Design review of the part built by this model. Coordinates are the model's own, in mm. Face numbers are marked on the shaded views. A direction names the side the tool comes from. Coordinates: 2 decimals unless noted, no trailing zeros. Write each loop counter-clockwise with the first axis right and the second up, starting at its lowest first coordinate (ties: lowest second). Pieces come first, ordered by that corner, then holes. Notation, with made-up numbers: M 16,18.25 L 32,18.25 A28 cw 32,40.25 Z; hole C 46,21.25 d8. An arc over 180 degrees is marked long. Return JSON: item names as keys, results as strings. Group by question number.
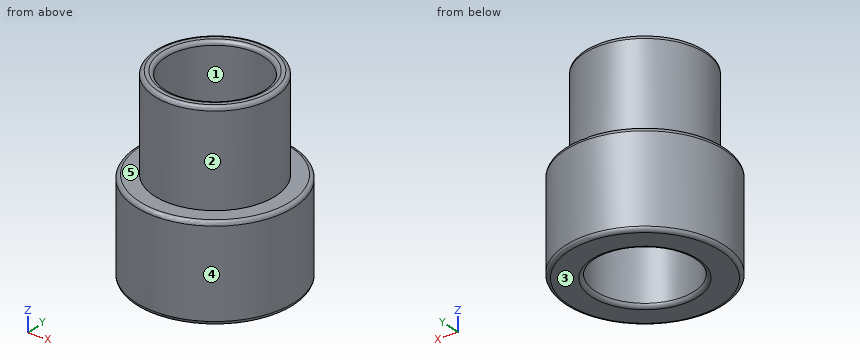
```python
from build123d import *

# Parameters (mm, degrees)
CYLINDER002_R     = 13
CYLINDER002_DEPTH = 120
CYLINDER001_R     = 16
CYLINDER001_DEPTH = 50
FILLET001_R       = 1
CYLINDER003_R     = 16
CYLINDER003_DEPTH = 120
CYLINDER_R        = 21
CYLINDER_DEPTH    = 25
FILLET_R          = 1


with BuildPart() as obj1:
    # Cylinder002 → Cylinder002 (new body)
    with BuildSketch(Plane.XY.offset(-60)):
        Circle(CYLINDER002_R)
    extrude(amount=CYLINDER002_DEPTH)


with BuildPart() as fillet001:
    # Cylinder001 → Cylinder001 (new body)
    with BuildSketch(Plane.XY):
        Circle(CYLINDER001_R)
    extrude(amount=CYLINDER001_DEPTH)

    # Cut: cut obj1
    add(obj1.part, mode=Mode.SUBTRACT)

    # Fillet001
    fillet001_edges = [fillet001.edges().sort_by_distance(p)[0] for p in [
        (-16, 0, 50),
        (-13, 0, 50),
        (-13, 0, 0),
    ]]
    fillet(fillet001_edges, radius=FILLET001_R)


with BuildPart() as obj2:
    # Cylinder003 → Cylinder003 (new body)
    with BuildSketch(Plane.XY.offset(-60)):
        Circle(CYLINDER003_R)
    extrude(amount=CYLINDER003_DEPTH)


with BuildPart() as fusion:
    # Cylinder → Cylinder (new body)
    with BuildSketch(Plane.XY):
        Circle(CYLINDER_R)
    extrude(amount=CYLINDER_DEPTH)

    # Cut001: cut obj2
    add(obj2.part, mode=Mode.SUBTRACT)

    # Fillet
    fillet_edges = [fusion.edges().sort_by_distance(p)[0] for p in [
        (-21, 0, 25),
        (-21, 0, 0),
    ]]
    fillet(fillet_edges, radius=FILLET_R)

    # Fusion: union Fillet001
    add(fillet001.part)


solid = fusion.part
```
Item 1: For pin 1 (4 mm diameter, centred on y = -11.5, z = 30.5, fed in from +X); pin 2 (12 mm diameter, centred on x = 2, y = 4, fed in from +Z); pin 3 (5 mm diameter, centred on x = -16.5, y = -15, fed in from +Z); pin 4 (1.5 mm diameter, centred on y = -1.5, z = 41, fed in from +X), all flat-tipped, find the tip position at first contact; note any pin that passes through.
Item 2: Add section A-A (x = 0). Write out the cut boundary in (y, z).
Item 3: Machinability: for the marked faces 4 and 5, which of the approach directions +Z, -Z, +X, -X, +Y, -Y give a long, thin tool a straight path to every point of the face, cutting with its end or side? Answer none if there is none.
Item 4: The part is to be moulded in two halves that separate along Y. For the marked faces 1, 2 and 3, say which applies: pulls with the +Y half, pulls with the -Y half, needs draft (parallel to the pull), parting line crosses it, or undercut.
Item 5: For line 1 (Y direction, x = 0, z = 36); line 2 (Y direction, x = 0, z = 22), list the stretches that pass through material, from the lowest coordinate up.
Item 6: Add section C-C (z = 34.5). Write out the cut boundary in (x, y), plus the area to 3 significant figures.
Geometry check:
{
 "1": {"pin 1": "x = 12.87", "pin 2": "through", "pin 3": "z = 25", "pin 4": "x = 15.98"},
 "2": {"outline": "M -21,1 A1 ccw -20,0 L -14,0 A1 ccw -13,1 L -13,49 A1 ccw -14,50 L -15,50 A1 ccw -16,49 L -16,25 L -20,25 A1 ccw -21,24 Z; M 13,1 A1 ccw 14,0 L 20,0 A1 ccw 21,1 L 21,24 A1 ccw 20,25 L 16,25 L 16,49 A1 ccw 15,50 L 14,50 A1 ccw 13,49 Z"},
 "3": {"face 4": "+Z, -Z", "face 5": "+Z"},
 "4": {"face 1": "undercut", "face 2": "parting line crosses it", "face 3": "needs draft"},
 "5": {"line 1": "-16 to -13, 13 to 16", "line 2": "-21 to -13, 13 to 21"},
 "6": {"outline": "C 0,0 d32; hole C 0,0 d26", "area": "273 mm^2"}
}
